Source: CAD feature listing. Evaluate the final solid. Frame: model axes, mm. A direction names the side the tool comes from. Give positions to 0.01 mm unless a question says otherwise; leave off trailing zeros. Order: outer loops, then holes, each group sorted by start corner. A loop starts at its lowest first (then second) coordinate and runs counter-clockwise, first axis right, second up. Notation, with made-up numbers: (19, 78.25) - (33, 78.25) arc R20 cw to (33, 104.25) - close; hole circle Ø5 at (59.25, -9.5). An arc over 180 degrees is marked (long way). Answer as CSV lines item,"result".
```python
from build123d import *

# Parameters (mm, degrees)
F1_DEPTH     = 30
F3_DEPTH     = 1000
F5_DEPTH     = 25
F6_W         = 5
F6_H         = 408.0812203564
F7_DEPTH     = 400
F8_T4_DEPTH  = 1805.1780915761
F8_T10_DEPTH = 1805.1780915761
F8_T16_DEPTH = 1805.1780915761
F8_T22_DEPTH = 1805.1780915761
F8_T28_DEPTH = 1805.1780915761
F8_T34_DEPTH = 1805.1780915761
F8_T40_DEPTH = 1805.1780915761
F8_T46_DEPTH = 1805.1780915761
F8_T52_DEPTH = 1805.1780915761
F8_T58_DEPTH = 1805.1780915761
F8_T64_DEPTH = 1805.1780915761
F8_T70_DEPTH = 1805.1780915761
F12_DEPTH    = 30
F13_DEPTH    = 5


# Not quite as in the source:
# - a fillet or chamfer that OpenCascade refuses, or shapes differently, is made with other operations: its cross-section is extruded or revolved along the edge and cut away or added


with BuildPart() as f1:
    # F0 (on Top) → F1 (new body)
    with BuildSketch(Plane.XY):
        Polygon((-190, 550), (-550, 550), (-550, -130), (-330, -350), (350, -350), (350, 10), (-180.8831175457, 10), (-190, 19.1168824543), align=None)
    extrude(amount=F1_DEPTH)

    # F2 (on face) → F3 (join)
    with BuildSketch(Plane(origin=(0, 0, 0), x_dir=(1, 0, 0), z_dir=(0, 0, -1))):
        Polygon((-330, 350), (-550, 130), (-190, -19.1168824543), (-180.8831175457, -10), align=None)
    extrude(amount=F3_DEPTH)

    # F4 (on face) → F5 (join)
    with BuildSketch(Plane(origin=(0, 0, -1000), x_dir=(1, 0, 0), z_dir=(0, 0, -1))):
        Polygon((350, 350), (-330, 350), (-550, 130), (-550, -550), (-190, -550), (-190, -19.1168824543), (-180.8831175457, -10), (350, -10), align=None)
    extrude(amount=F5_DEPTH)

    # F6 (on face) → F7 (join)
    with BuildSketch(Plane(origin=(0, 0, 0), x_dir=(1, 0, 0), z_dir=(0, 0, -1))):
        Polygon((-311.3603896932, 305), (94.6497628513, 305), (94.6497628513, 310), (-313.4314575051, 310), align=None)
        with Locations((-507.5, -90.6091526731)):
            Rectangle(F6_W, F6_H)
        Polygon((94.6497628513, 30), (94.6497628513, 35), (-199.5227278525, 35), (-197.4516600406, 30), align=None)
        Polygon((-235, -0.4772721475), (-235, -294.6497628513), (-230, -294.6497628513), (-230, -2.5483399594), align=None)
    extrude(amount=F7_DEPTH)

    # F8: chamfer of 350 on 4 edges, made by hand


with BuildPart() as f8_tool2:
    # F8_s3 → F8_t4 (new body)
    with BuildSketch(Plane.YZ.offset(-1410.0890457881)):
        Polygon((-55.3502371487, -400), (294.6497628513, -50), (294.6497628513, -400), align=None)
    extrude(amount=F8_T4_DEPTH)

    split(bisect_by=Plane(origin=(-34.5836943966, 83.4924240492, 0), x_dir=(0, 0, 1), z_dir=(-0.3826834324, 0.9238795325, 0)), keep=Keep.TOP)

    split(bisect_by=Plane(origin=(-157.9289321881, 65.4163056034, 0), x_dir=(0, 0, 1), z_dir=(-0.9238795325, 0.3826834324, 0)), keep=Keep.TOP)


with BuildPart() as f1_1:
    add(f1.part)

    # F8_t1: cut F8_tool2
    add(f8_tool2.part, mode=Mode.SUBTRACT)


with BuildPart() as f8_tool8:
    # F8_s9 → F8_t10 (new body)
    with BuildSketch(Plane.YZ.offset(-1410.0890457881)):
        Polygon((-55.3502371487, -400), (294.6497628513, -50), (294.6497628513, -400), align=None)
    extrude(amount=F8_T10_DEPTH)

    split(bisect_by=Plane(origin=(-34.5836943966, 83.4924240492, 0), x_dir=(0, 0, 1), z_dir=(-0.3826834324, 0.9238795325, 0)), keep=Keep.TOP)

    split(bisect_by=Plane(origin=(-157.9289321881, 65.4163056034, 0), x_dir=(0, 0, 1), z_dir=(0.9238795325, -0.3826834324, 0)), keep=Keep.TOP)


with BuildPart() as f1_2:
    add(f1_1.part)

    # F8_t7: cut F8_tool8
    add(f8_tool8.part, mode=Mode.SUBTRACT)


with BuildPart() as f8_tool14:
    # F8_s15 → F8_t16 (new body)
    with BuildSketch(Plane.YZ.offset(-1410.0890457881)):
        Polygon((-55.3502371487, -400), (294.6497628513, -50), (294.6497628513, -400), align=None)
    extrude(amount=F8_T16_DEPTH)

    split(bisect_by=Plane(origin=(-34.5836943966, 83.4924240492, 0), x_dir=(0, 0, 1), z_dir=(0.3826834324, -0.9238795325, 0)), keep=Keep.TOP)

    split(bisect_by=Plane(origin=(-157.9289321881, 65.4163056034, 0), x_dir=(0, 0, 1), z_dir=(0.9238795325, -0.3826834324, 0)), keep=Keep.TOP)


with BuildPart() as f1_3:
    add(f1_2.part)

    # F8_t13: cut F8_tool14
    add(f8_tool14.part, mode=Mode.SUBTRACT)


with BuildPart() as f8_tool20:
    # F8_s21 → F8_t22 (new body)
    with BuildSketch(Plane.XZ.offset(-595.0890457881)):
        Polygon((-255.3502371487, -400), (94.6497628513, -50), (94.6497628513, -400), align=None)
    extrude(amount=F8_T22_DEPTH)

    split(bisect_by=Plane(origin=(-34.5836943966, 83.4924240492, 0), x_dir=(0, 0, 1), z_dir=(-0.3826834324, 0.9238795325, 0)), keep=Keep.TOP)

    split(bisect_by=Plane(origin=(-157.9289321881, 65.4163056034, 0), x_dir=(0, 0, 1), z_dir=(-0.9238795325, 0.3826834324, 0)), keep=Keep.TOP)


with BuildPart() as f1_4:
    add(f1_3.part)

    # F8_t19: cut F8_tool20
    add(f8_tool20.part, mode=Mode.SUBTRACT)


with BuildPart() as f8_tool26:
    # F8_s27 → F8_t28 (new body)
    with BuildSketch(Plane.XZ.offset(-595.0890457881)):
        Polygon((-255.3502371487, -400), (94.6497628513, -50), (94.6497628513, -400), align=None)
    extrude(amount=F8_T28_DEPTH)

    split(bisect_by=Plane(origin=(-34.5836943966, 83.4924240492, 0), x_dir=(0, 0, 1), z_dir=(-0.3826834324, 0.9238795325, 0)), keep=Keep.TOP)

    split(bisect_by=Plane(origin=(-157.9289321881, 65.4163056034, 0), x_dir=(0, 0, 1), z_dir=(0.9238795325, -0.3826834324, 0)), keep=Keep.TOP)


with BuildPart() as f1_5:
    add(f1_4.part)

    # F8_t25: cut F8_tool26
    add(f8_tool26.part, mode=Mode.SUBTRACT)


with BuildPart() as f8_tool32:
    # F8_s33 → F8_t34 (new body)
    with BuildSketch(Plane.XZ.offset(-595.0890457881)):
        Polygon((-255.3502371487, -400), (94.6497628513, -50), (94.6497628513, -400), align=None)
    extrude(amount=F8_T34_DEPTH)

    split(bisect_by=Plane(origin=(-34.5836943966, 83.4924240492, 0), x_dir=(0, 0, 1), z_dir=(0.3826834324, -0.9238795325, 0)), keep=Keep.TOP)

    split(bisect_by=Plane(origin=(-157.9289321881, 65.4163056034, 0), x_dir=(0, 0, 1), z_dir=(0.9238795325, -0.3826834324, 0)), keep=Keep.TOP)


with BuildPart() as f1_6:
    add(f1_5.part)

    # F8_t31: cut F8_tool32
    add(f8_tool32.part, mode=Mode.SUBTRACT)


with BuildPart() as f8_tool38:
    # F8_s39 → F8_t40 (new body)
    with BuildSketch(Plane.YZ.offset(-1135.0890457881)):
        Polygon((-55.3502371487, -400), (294.6497628513, -50), (294.6497628513, -400), align=None)
    extrude(amount=F8_T40_DEPTH)

    split(bisect_by=Plane(origin=(-34.5836943966, 83.4924240492, 0), x_dir=(0, 0, 1), z_dir=(-0.3826834324, 0.9238795325, 0)), keep=Keep.TOP)

    split(bisect_by=Plane(origin=(-157.9289321881, 65.4163056034, 0), x_dir=(0, 0, 1), z_dir=(-0.9238795325, 0.3826834324, 0)), keep=Keep.TOP)


with BuildPart() as f1_7:
    add(f1_6.part)

    # F8_t37: cut F8_tool38
    add(f8_tool38.part, mode=Mode.SUBTRACT)


with BuildPart() as f8_tool44:
    # F8_s45 → F8_t46 (new body)
    with BuildSketch(Plane.YZ.offset(-1135.0890457881)):
        Polygon((-55.3502371487, -400), (294.6497628513, -50), (294.6497628513, -400), align=None)
    extrude(amount=F8_T46_DEPTH)

    split(bisect_by=Plane(origin=(-34.5836943966, 83.4924240492, 0), x_dir=(0, 0, 1), z_dir=(-0.3826834324, 0.9238795325, 0)), keep=Keep.TOP)

    split(bisect_by=Plane(origin=(-157.9289321881, 65.4163056034, 0), x_dir=(0, 0, 1), z_dir=(0.9238795325, -0.3826834324, 0)), keep=Keep.TOP)


with BuildPart() as f1_8:
    add(f1_7.part)

    # F8_t43: cut F8_tool44
    add(f8_tool44.part, mode=Mode.SUBTRACT)


with BuildPart() as f8_tool50:
    # F8_s51 → F8_t52 (new body)
    with BuildSketch(Plane.YZ.offset(-1135.0890457881)):
        Polygon((-55.3502371487, -400), (294.6497628513, -50), (294.6497628513, -400), align=None)
    extrude(amount=F8_T52_DEPTH)

    split(bisect_by=Plane(origin=(-34.5836943966, 83.4924240492, 0), x_dir=(0, 0, 1), z_dir=(0.3826834324, -0.9238795325, 0)), keep=Keep.TOP)

    split(bisect_by=Plane(origin=(-157.9289321881, 65.4163056034, 0), x_dir=(0, 0, 1), z_dir=(0.9238795325, -0.3826834324, 0)), keep=Keep.TOP)


with BuildPart() as f1_9:
    add(f1_8.part)

    # F8_t49: cut F8_tool50
    add(f8_tool50.part, mode=Mode.SUBTRACT)


with BuildPart() as f8_tool56:
    # F8_s57 → F8_t58 (new body)
    with BuildSketch(Plane.XZ.offset(-870.0890457881)):
        Polygon((-255.3502371487, -400), (94.6497628513, -50), (94.6497628513, -400), align=None)
    extrude(amount=F8_T58_DEPTH)

    split(bisect_by=Plane(origin=(-34.5836943966, 83.4924240492, 0), x_dir=(0, 0, 1), z_dir=(-0.3826834324, 0.9238795325, 0)), keep=Keep.TOP)

    split(bisect_by=Plane(origin=(-157.9289321881, 65.4163056034, 0), x_dir=(0, 0, 1), z_dir=(-0.9238795325, 0.3826834324, 0)), keep=Keep.TOP)


with BuildPart() as f1_10:
    add(f1_9.part)

    # F8_t55: cut F8_tool56
    add(f8_tool56.part, mode=Mode.SUBTRACT)


with BuildPart() as f8_tool62:
    # F8_s63 → F8_t64 (new body)
    with BuildSketch(Plane.XZ.offset(-870.0890457881)):
        Polygon((-255.3502371487, -400), (94.6497628513, -50), (94.6497628513, -400), align=None)
    extrude(amount=F8_T64_DEPTH)

    split(bisect_by=Plane(origin=(-34.5836943966, 83.4924240492, 0), x_dir=(0, 0, 1), z_dir=(-0.3826834324, 0.9238795325, 0)), keep=Keep.TOP)

    split(bisect_by=Plane(origin=(-157.9289321881, 65.4163056034, 0), x_dir=(0, 0, 1), z_dir=(0.9238795325, -0.3826834324, 0)), keep=Keep.TOP)


with BuildPart() as f1_11:
    add(f1_10.part)

    # F8_t61: cut F8_tool62
    add(f8_tool62.part, mode=Mode.SUBTRACT)


with BuildPart() as f8_tool68:
    # F8_s69 → F8_t70 (new body)
    with BuildSketch(Plane.XZ.offset(-870.0890457881)):
        Polygon((-255.3502371487, -400), (94.6497628513, -50), (94.6497628513, -400), align=None)
    extrude(amount=F8_T70_DEPTH)

    split(bisect_by=Plane(origin=(-34.5836943966, 83.4924240492, 0), x_dir=(0, 0, 1), z_dir=(0.3826834324, -0.9238795325, 0)), keep=Keep.TOP)

    split(bisect_by=Plane(origin=(-157.9289321881, 65.4163056034, 0), x_dir=(0, 0, 1), z_dir=(0.9238795325, -0.3826834324, 0)), keep=Keep.TOP)


with BuildPart() as f1_12:
    add(f1_11.part)

    # F8_t67: cut F8_tool68
    add(f8_tool68.part, mode=Mode.SUBTRACT)

    # F11 (on face) → F12 (cut, through all)
    with BuildSketch(Plane.XY.offset(30)):
        Polygon((-431.5, -80.9156928588), (-280.9156928588, -231.5), (350, -231.5), (350, -228.5), (-279.6730521717, -228.5), (-428.5, -79.6730521717), (-428.5, 550), (-431.5, 550), align=None)
        Polygon((-311.5, -31.210065374), (-231.210065374, -111.5), (350, -111.5), (350, -108.5), (-229.9674246869, -108.5), (-308.5, -29.9674246869), (-308.5, 550), (-311.5, 550), align=None)
    extrude(amount=-F12_DEPTH, mode=Mode.SUBTRACT)

    # F9 (on face) → F13 (join)
    with BuildSketch(Plane(origin=(0, 0, 0), x_dir=(1, 0, 0), z_dir=(0, 0, -1))):
        Polygon((94.6497628513, 255), (94.6497628513, 305), (-311.3603896932, 305), (-290.6497115746, 255), (44.6497628513, 255), (44.6497628513, 85), (-220.2334059711, 85), (-199.5227278525, 35), (94.6497628513, 35), (94.6497628513, 85), align=None)
        Polygon((-285, -294.6497628513), (-235, -294.6497628513), (-235, -0.4772721475), (-285, 20.2334059711), (-285, -244.6497628513), (-455, -244.6497628513), (-455, 90.6497115746), (-505, 111.3603896932), (-505, -294.6497628513), (-455, -294.6497628513), align=None)
    extrude(amount=F13_DEPTH)


solid = f1_12.part
```
(1) Mould query, pull axis X, two halves, no side actions, for faces 4 (the flat face through (-550, 215, 15)), 5 (the flat face through (-190, 281, 15)), 6 (the flat face through (-369, 550, 15)), 7 (the flat face through (-505, 49, -156)). Classes: released by +X, released by -X, zero draft, split by the parting line, or undercut.
Completed:
face 4,"released by -X"
face 5,"released by +X"
face 6,"zero draft"
face 7,"undercut"
(2) Cut plane A-A (y = 414.5). Return loops of the section in (x, z).
Completed:
outline,"(-550, -1025) - (-190, -1025) - (-190, -1000) - (-550, -1000) - close; (-550, 0) - (-431.5, 0) - (-431.5, 30) - (-550, 30) - close; (-428.5, 0) - (-311.5, 0) - (-311.5, 30) - (-428.5, 30) - close; (-308.5, 0) - (-190, 0) - (-190, 30) - (-308.5, 30) - close"
(3) Contact query for flat-ended pins moving along their axis: pin 1 (2 mm diameter, centred on x = -271.5, z = -839, fed in from -Y); pin 2 (4 mm diameter, centred on x = -424, z = -903, fed in from -Y); pin 3 (3 mm diameter, centred on x = -404.5, z = -731, fed in from -Y). Output: stop coordinate, or through.
Completed:
pin 1,"y = -211.18"
pin 2,"y = -258"
pin 3,"y = -277"
(4) Cut plane D-D (z = -822). Return loops of the section in (x, y), then the cut area to 3 significant figures.
Completed:
outline,"(-550, -130) - (-330, -350) - (-180.88, 10) - (-190, 19.12) - close"
area,"58,300 mm²"
(5) Access query for faces 1 (the flat face through (-83, -35, -135)), 2 (the flat face through (88, 10, 15)), 3 (the flat face through (-120, -169, 0)). Directions: +Z, -Z, +X, -X, +Y, -Y. A direction counts if a zero-diameter tool reaches every point of the face in a straight line with its end or side. Return the directions, or none.
Completed:
face 1,"+X"
face 2,"+Z, -Z, +X, +Y"
face 3,"none"
(6) Cut plane B-B (x = 67). Return loops of the section in (y, z).
Completed:
outline,"(-350, -1025) - (10, -1025) - (10, -1000) - (-350, -1000) - close; (-350, 0) - (-310, 0) - (-310, -77.65) - (-305, -77.65) - (-305, -5) - (-35, -5) - (-35, -77.65) - (-30, -77.65) - (-30, 0) - (10, 0) - (10, 30) - (-108.5, 30) - (-108.5, 0) - (-111.5, 0) - (-111.5, 30) - (-228.5, 30) - (-228.5, 0) - (-231.5, 0) - (-231.5, 30) - (-350, 30) - close"
(7) Cut plane C-C (x = -117.5). Return loops of the section in (y, z), then the cut area to 3 significant figures.
Completed:
outline,"(-350, -1025) - (10, -1025) - (10, -1000) - (-350, -1000) - close; (-350, 0) - (-310, 0) - (-310, -262.15) - (-305, -262.15) - (-305, -5) - (-255, -5) - (-255, 0) - (-231.5, 0) - (-231.5, 30) - (-350, 30) - close; (-228.5, 0) - (-111.5, 0) - (-111.5, 30) - (-228.5, 30) - close; (-108.5, 0) - (-85, 0) - (-85, -5) - (-35, -5) - (-35, -262.15) - (-30, -262.15) - (-30, 0) - (10, 0) - (10, 30) - (-108.5, 30) - close"
area,"22,700 mm²"
(8) Ray query, line 1 (Z direction, x = 129.5, y = -16.5); line 2 (Z direction, x = -489, y = -55); line 3 (Y direction, x = -205, z = -34.5). Return the intervals inside material, ascending. Write a range as from..to.
Completed:
line 1,"-1025..-1000, 0..30"
line 2,"-1025..-1000, -5..30"
line 3,"-310..-305, -48.22..12.9"
